```python
from build123d import *

# Parameters (mm, degrees)
SKETCH1_W           = 35
SKETCH1_H           = 10
BOSS_EXTRUDE1_DEPTH = 60.5
SKETCH2_R           = 11
CUT_EXTRUDE1_DEPTH  = 11
SKETCH3_R           = 1.75
CUT_EXTRUDE2_DEPTH  = 10
FILLET1_R           = 12
SKETCH4_R           = 12.7
CUT_EXTRUDE3_DEPTH  = 4


with BuildPart() as part:
    # Sketch1 → Boss-Extrude1 (new body)
    with BuildSketch(Plane(origin=(0, 0, 0), x_dir=(1, 0, 0), z_dir=(0, 1, 0))):
        with Locations((1.164675851, 0)):
            Rectangle(SKETCH1_W, SKETCH1_H)
    extrude(amount=BOSS_EXTRUDE1_DEPTH)

    # Sketch2 → Cut-Extrude1 (cut, through all)
    with BuildSketch(Plane.XY.offset(5)):
        with Locations((1.164675851, 45.5)):
            Circle(SKETCH2_R)
    extrude(amount=-CUT_EXTRUDE1_DEPTH, mode=Mode.SUBTRACT)

    # Sketch3 → Cut-Extrude2 (cut)
    with BuildSketch(Plane.XZ):
        with Locations((-8.335324149, 0)):
            Circle(SKETCH3_R)
        with Locations((10.664675851, 0)):
            Circle(SKETCH3_R)
    extrude(amount=-CUT_EXTRUDE2_DEPTH, mode=Mode.SUBTRACT)

    # Fillet1
    fillet1_edges = [part.edges().sort_by_distance(p)[0] for p in [
        (18.664675851, 60.5, 0),
        (-16.335324149, 60.5, 0),
    ]]
    fillet(fillet1_edges, radius=FILLET1_R)

    # Sketch4 → Cut-Extrude3 (cut)
    with BuildSketch(Plane.XY.offset(5)):
        with Locations((1.164675851, 45.5)):
            Circle(SKETCH4_R)
    extrude(amount=-CUT_EXTRUDE3_DEPTH, mode=Mode.SUBTRACT)


solid = part.part
```
CAD build for the part. Positions are in the model's coordinates, mm. A direction names the side the tool comes from. Coordinates: 2 decimals unless noted, no trailing zeros. Loops run counter-clockwise (first coordinate to the right, second up) from the corner with the lowest first, then second, coordinate; pieces in that order, holes last. Notation, with made-up numbers: (46.5, 87) - (99.5, 87) arc R17 cw to (99.5, 117) - close; hole circle Ø8 at (-36, 63). An arc over 180 degrees is marked (long way). Use CSV: the item, a comma, the result in double quotes. Start each with the question number.
Q1. Cut at B-B, the plane z = -2.5. List the corners of the cut face in (x, y), then the cut area to 3 significant figures.
Q2. Cut at A-A, the plane y = 45.5. List the corners of the cut face in (x, z).
Q3. Drop flat-ended pins along their axis: P1, Ø1, axis at x = -8.5, z = 0.5, coming from the -Y side; P2, Ø2, axis at x = -8.34, z = 0, coming from the +Y side. Give the stop position or say it passes through.
Q4. Probe probe 1 along Y at (x, z) = (9, 3); probe 2 along Y at (x, z) = (11, -1.5); probe 3 along X at (y, z) = (35, 4.5). List the from-to ranges inside material, lowest first. Write a range as from..to.
Q5. Cut at C-C, the plane x = 1.5. List the corners of the cut face in (y, z).
Q6. 3-axis set-ups, long thin cutter, end or side, ignore diameter. For faces 1 (the flat face through (-16.335, 24, 0)), 2 (the cylindrical face through (13.28, 49.31, 3.03)), 3 (the cylindrical face through (-10.084, 4.93, 0.077)): which of +Z, -Z, +X, -X, +Y, -Y reach the whole face in a straight line?
Q7. Two-plate mould, pull along Z, no slides. Class faces 4 (the cylindrical face through (15.056, 57.078, -0.07)), 5 (the flat face through (11, 10, 0)), 6 (the flat face through (1, 23, -5)), 7 (the flat face through (-3, 56, 1)): +Z half, -Z half, draft (parallel to the pull), parting line (faces both ways), or undercut.
Q8. Cut at D-D, the plane z = 0. List the corners of the cut face in (x, y), then the cut area to 3 significant figures.
Here are the results:
1,outline,"(-16.34, 0) - (18.66, 0) - (18.66, 48.5) arc R12 ccw to (6.66, 60.5) - (-4.34, 60.5) arc R12 ccw to (-16.34, 48.5) - close; hole circle Ø22 at (1.16, 45.5)"
1,area,"1,680 mm2"
2,outline,"(-16.34, -5) - (-9.84, -5) - (-9.84, 1) - (-11.54, 1) - (-11.54, 5) - (-16.34, 5) - close; (12.16, -5) - (18.66, -5) - (18.66, 5) - (13.86, 5) - (13.86, 1) - (12.16, 1) - close"
3,P1,"y = 10"
3,P2,"y = 60.12"
4,probe 1,"0..35.51, 55.49..60.27"
4,probe 2,"10..40.57, 50.43..59.69"
4,probe 3,"-16.34..-5.98, 8.31..18.66"
5,outline,"(0, -5) - (34.51, -5) - (34.51, 1) - (32.8, 1) - (32.8, 5) - (0, 5) - close; (56.49, -5) - (60.5, -5) - (60.5, 5) - (58.2, 5) - (58.2, 1) - (56.49, 1) - close"
6,face 1,"+Z, -Z, -X, +Y, -Y"
6,face 2,"+Z"
6,face 3,"-Y"
7,face 4,"draft"
7,face 5,"undercut"
7,face 6,"-Z half"
7,face 7,"+Z half"
8,outline,"(-16.34, 0) - (-10.09, 0) - (-10.09, 10) - (-6.59, 10) - (-6.59, 0) - (8.91, 0) - (8.91, 10) - (12.41, 10) - (12.41, 0) - (18.66, 0) - (18.66, 48.5) arc R12 ccw to (6.66, 60.5) - (-4.34, 60.5) arc R12 ccw to (-16.34, 48.5) - close; hole circle Ø22 at (1.16, 45.5)"
8,area,"1,610 mm2"
